Here's how the part is built. I have some questions about the finished solid (model axes, mm). A direction names the side the tool comes from. Coordinates: 2 decimals unless noted, no trailing zeros. Loops run counter-clockwise (first coordinate to the right, second up) from the corner with the lowest first, then second, coordinate; pieces in that order, holes last. Notation, with made-up numbers: (-28.5, 40) -> (22.5, 40) arc R31 ccw to (22.5, 79) -> close; hole circle Ø5 at (7.5, 23). An arc over 180 degrees is marked (long way). Answer as a JSON object with one key per item and string values. Group by question number.
Q1. I need wall thicknesses on line 1 (Z direction, x = -30.5, y = 95); line 2 (Z direction, x = 55, y = 8); line 3 (X direction, y = 60, z = 31.5). Which ranges of each line are inside material? Lowest first, please.
Q2. I want a section at C-C on z = 82.5. Write out the boundary of the cut face in (x, y).
Q3. I want a section at D-D on x = 43.5. Write out the boundary of the cut face in (y, z).
Q4. I'm going to push flat-ended pins straight in: pin 1 (0.8 mm diameter, centred on x = 24, z = 64, fed in from -Y); pin 2 (1.2 mm diameter, centred on x = 99.5, y = 43.5, fed in from +Z); pin 3 (1 mm diameter, centred on x = -36, y = 77, fed in from +Z); pin 4 (1 mm diameter, centred on x = 52, z = 55, fed in from +Y). Where does each tip first touch, or does it pass through?
Q5. On a 3-axis mill with a long thin cutter (end or side, diameter ignored), from which of +Z, -Z, +X, -X, +Y, -Y can I reach the whole of each face in a straight line? I mean faces 1 (the flat face through (-37, 94, 98.5)), 2 (the flat face through (-1, 0, -1)). Say none if no direction works.
Q6. Thinking about a two-plate mould opening in Y: for faces 3 (the flat face through (-100, 92, -2)), 4 (the flat face through (1.4, 149.375, -107.083)), 5 (the flat face through (61, 78, 30)), 6 (the flat face through (1.4, 169.1, -58)), which applies, released by +Y, released by -Y, zero draft, split by the parting line, or undercut?
Q7. I want a section at B-B on x = 71. Write out the boundary of the cut face in (y, z), then the cut area to 3 significant figures.
```python
from build123d import *

# Parameters (mm, degrees)
SKETCH_1_W           = 150
SKETCH_1_H           = 3.5
EXTRUDE_1_DEPTH      = 1.5
SKETCH_2_W           = 121.171669679
SKETCH_2_H           = 150
EXTRUDE_2_DEPTH      = 91.5
SKETCH_3_W           = 1.5
SKETCH_3_H           = 90
EXTRUDE_3_DEPTH      = 30
EXTRUDE_4_DEPTH      = 30
SKETCH_5_W           = 151.171669679
SKETCH_5_H           = 125
EXTRUDE_5_DEPTH      = 1.5
SKETCH_6_W           = 125
SKETCH_6_H           = 151.5
EXTRUDE_6_DEPTH      = 48.828330321
SKETCH_7_W           = 200
SKETCH_7_H           = 151.5
EXTRUDE_7_DEPTH      = 75
SKETCH_8_W           = 74.671669679
SKETCH_8_H           = 150
CUT_EXTRUDE_1_DEPTH  = 53.5
SKETCH_9_W           = 30
SKETCH_9_H           = 150
CUT_EXTRUDE_2_DEPTH  = 59.25
SKETCH_10_W          = 59.25
SKETCH_10_H          = 150
CUT_EXTRUDE_3_DEPTH  = 42.671669679
SKETCH_11_W          = 30
SKETCH_11_H          = 60
CUT_EXTRUDE_4_DEPTH  = 1.5
SKETCH_12_W          = 30
SKETCH_12_H          = 60
CUT_EXTRUDE_5_DEPTH  = 1.5
SKETCH_13_W          = 87
SKETCH_13_H          = 150
CUT_EXTRUDE_6_DEPTH  = 47.328330321
SKETCH_14_W          = 59.25
SKETCH_14_H          = 150
CUT_EXTRUDE_7_DEPTH  = 47.328330321
SKETCH_15_W          = 120
SKETCH_15_H          = 150
CUT_EXTRUDE_8_DEPTH  = 29.25
SKETCH_16_W          = 88.5
SKETCH_16_H          = 150
CUT_EXTRUDE_9_DEPTH  = 75.5
SKETCH_17_W          = 122
SKETCH_17_H          = 150
CUT_EXTRUDE_10_DEPTH = 20
SKETCH_18_W          = 50
SKETCH_18_H          = 150
CUT_EXTRUDE_11_DEPTH = 73.5
SKETCH_19_W          = 73.5
SKETCH_19_H          = 150
CUT_EXTRUDE_12_DEPTH = 18.5
SKETCH_20_W          = 75
SKETCH_20_H          = 150
CUT_EXTRUDE_13_DEPTH = 3.5
CUT_EXTRUDE_14_REACH = 272.097
SKETCH_21_W          = 30
SKETCH_21_H          = 30
CUT_EXTRUDE_15_REACH = 272.097
SKETCH_22_W          = 30
SKETCH_22_H          = 30
CUT_EXTRUDE_16_REACH = 272.097
SKETCH_23_W          = 30
SKETCH_23_H          = 30
EXTRUDE_11_DEPTH     = 200
EXTRUDE_12_DEPTH     = 200


with BuildPart() as part:
    # Sketch 1 → Extrude 1 (new body)
    with BuildSketch(Plane(origin=(98.5, 0, 0), x_dir=(0, -1, 0), z_dir=(-1, 0, 0))):
        with Locations((-76.5, -6.75)):
            Rectangle(SKETCH_1_W, SKETCH_1_H)
    extrude(amount=-EXTRUDE_1_DEPTH)

    # Sketch 2 → Extrude 2 (add)
    with BuildSketch(Plane(origin=(0, 0, -8.5), x_dir=(-1, 0, 0), z_dir=(0, 0, -1))):
        with Locations((-39.41416516, 76.5)):
            Rectangle(SKETCH_2_W, SKETCH_2_H)
    extrude(amount=EXTRUDE_2_DEPTH)

    # Sketch 3 → Extrude 3 (add)
    with BuildSketch(Plane.XY.offset(-5)):
        with Locations((99.25, 106.5)):
            Rectangle(SKETCH_3_W, SKETCH_3_H)
    extrude(amount=EXTRUDE_3_DEPTH)

    # Sketch 4 → Extrude 4 (add)
    with BuildSketch(Plane.ZY.offset(21.171669679)):
        Polygon((-100, 1.5), (-100, 151.5), (-8.5, 151.5), (-8.5, 61.5), (-10, 61.5), (-10, 1.5), align=None)
    extrude(amount=EXTRUDE_4_DEPTH)

    # Sketch 5 → Extrude 5 (add)
    with BuildSketch(Plane.XZ.offset(-1.5)):
        with Locations((24.41416516, -37.5)):
            Rectangle(SKETCH_5_W, SKETCH_5_H)
    extrude(amount=EXTRUDE_5_DEPTH)

    # Sketch 6 → Extrude 6 (add)
    with BuildSketch(Plane.ZY.offset(51.171669679)):
        with Locations((-37.5, 75.75)):
            Rectangle(SKETCH_6_W, SKETCH_6_H)
    extrude(amount=EXTRUDE_6_DEPTH)

    # Sketch 7 → Extrude 7 (add)
    with BuildSketch(Plane.XY.offset(25)):
        with Locations((0, 75.75)):
            Rectangle(SKETCH_7_W, SKETCH_7_H)
    extrude(amount=EXTRUDE_7_DEPTH)

    # Sketch 8 → Cut-Extrude 1 (cut)
    with BuildSketch(Plane(origin=(0, 0, 25), x_dir=(-1, 0, 0), z_dir=(0, 0, -1))):
        with Locations((13.83583484, 76.5)):
            Rectangle(SKETCH_8_W, SKETCH_8_H)
    extrude(amount=-CUT_EXTRUDE_1_DEPTH, mode=Mode.SUBTRACT)

    # Sketch 9 → Cut-Extrude 2 (cut)
    with BuildSketch(Plane.XY.offset(-10)):
        with Locations((-36.171669679, 76.5)):
            Rectangle(SKETCH_9_W, SKETCH_9_H)
    extrude(amount=-CUT_EXTRUDE_2_DEPTH, mode=Mode.SUBTRACT)

    # Sketch 10 → Cut-Extrude 3 (cut)
    with BuildSketch(Plane.ZY.offset(21.171669679)):
        with Locations((-39.625, 76.5)):
            Rectangle(SKETCH_10_W, SKETCH_10_H)
    extrude(amount=-CUT_EXTRUDE_3_DEPTH, mode=Mode.SUBTRACT)

    # Sketch 11 → Cut-Extrude 4 (cut)
    with BuildSketch(Plane.ZY.offset(-23.5)):
        with Locations((63.5, 31.5)):
            Rectangle(SKETCH_11_W, SKETCH_11_H)
    extrude(amount=-CUT_EXTRUDE_4_DEPTH, mode=Mode.SUBTRACT)

    # Sketch 12 → Cut-Extrude 5 (cut)
    with BuildSketch(Plane.ZY.offset(-21.5)):
        with Locations((-54.25, 31.5)):
            Rectangle(SKETCH_12_W, SKETCH_12_H)
    extrude(amount=-CUT_EXTRUDE_5_DEPTH, mode=Mode.SUBTRACT)

    # Sketch 13 → Cut-Extrude 6 (cut)
    with BuildSketch(Plane(origin=(-51.171669679, 0, 0), x_dir=(0, 0, -1), z_dir=(1, 0, 0))):
        with Locations((-35, 76.5)):
            Rectangle(SKETCH_13_W, SKETCH_13_H)
    extrude(amount=-CUT_EXTRUDE_6_DEPTH, mode=Mode.SUBTRACT)

    # Sketch 14 → Cut-Extrude 7 (cut)
    with BuildSketch(Plane(origin=(-51.171669679, 0, 0), x_dir=(0, 0, -1), z_dir=(1, 0, 0))):
        with Locations((39.625, 76.5)):
            Rectangle(SKETCH_14_W, SKETCH_14_H)
    extrude(amount=-CUT_EXTRUDE_7_DEPTH, mode=Mode.SUBTRACT)

    # Sketch 15 → Cut-Extrude 8 (cut)
    with BuildSketch(Plane.XY.offset(-69.25)):
        with Locations((-38.5, 76.5)):
            Rectangle(SKETCH_15_W, SKETCH_15_H)
    extrude(amount=-CUT_EXTRUDE_8_DEPTH, mode=Mode.SUBTRACT)

    # Sketch 16 → Cut-Extrude 9 (cut)
    with BuildSketch(Plane.ZY.offset(-23)):
        with Locations((-54.25, 76.5)):
            Rectangle(SKETCH_16_W, SKETCH_16_H)
    extrude(amount=-CUT_EXTRUDE_9_DEPTH, mode=Mode.SUBTRACT)

    # Sketch 17 → Cut-Extrude 10 (cut)
    with BuildSketch(Plane(origin=(0, 0, 78.5), x_dir=(-1, 0, 0), z_dir=(0, 0, -1))):
        with Locations((37.5, 76.5)):
            Rectangle(SKETCH_17_W, SKETCH_17_H)
    extrude(amount=-CUT_EXTRUDE_10_DEPTH, mode=Mode.SUBTRACT)

    # Sketch 18 → Cut-Extrude 11 (cut)
    with BuildSketch(Plane.ZY.offset(-25)):
        with Locations((73.5, 76.5)):
            Rectangle(SKETCH_18_W, SKETCH_18_H)
    extrude(amount=-CUT_EXTRUDE_11_DEPTH, mode=Mode.SUBTRACT)

    # Sketch 19 → Cut-Extrude 12 (cut)
    with BuildSketch(Plane.XY.offset(48.5)):
        with Locations((61.75, 76.5)):
            Rectangle(SKETCH_19_W, SKETCH_19_H)
    extrude(amount=-CUT_EXTRUDE_12_DEPTH, mode=Mode.SUBTRACT)

    # Sketch 20 → Cut-Extrude 13 (cut)
    with BuildSketch(Plane(origin=(0, 0, 25), x_dir=(-1, 0, 0), z_dir=(0, 0, -1))):
        with Locations((-61, 76.5)):
            Rectangle(SKETCH_20_W, SKETCH_20_H)
    extrude(amount=-CUT_EXTRUDE_13_DEPTH, mode=Mode.SUBTRACT)

    # Sketch 21 → Cut-Extrude 14 (cut, up to next)
    with BuildSketch(Plane(origin=(0, 0, -100), x_dir=(-1, 0, 0), z_dir=(0, 0, -1)), mode=Mode.PRIVATE) as cut_extrude_14_sk1:
        with Locations((-52.804007689, 60.155834385)):
            Rectangle(SKETCH_21_W, SKETCH_21_H)
    cut_extrude_14_tool1 = extrude(cut_extrude_14_sk1.sketch, amount=-CUT_EXTRUDE_14_REACH, mode=Mode.PRIVATE) & part.part
    add(cut_extrude_14_tool1.solids().sort_by_distance((52.804008, 60.155834, -100))[0], mode=Mode.SUBTRACT)

    # Sketch 22 → Cut-Extrude 15 (cut, up to next)
    with BuildSketch(Plane(origin=(0, 0, -100), x_dir=(-1, 0, 0), z_dir=(0, 0, -1)), mode=Mode.PRIVATE) as cut_extrude_15_sk1:
        with Locations((36.226594007, 60.594472186)):
            Rectangle(SKETCH_22_W, SKETCH_22_H)
    cut_extrude_15_tool1 = extrude(cut_extrude_15_sk1.sketch, amount=-CUT_EXTRUDE_15_REACH, mode=Mode.PRIVATE) & part.part
    add(cut_extrude_15_tool1.solids().sort_by_distance((-36.226594, 60.594472, -100))[0], mode=Mode.SUBTRACT)

    # Sketch 23 → Cut-Extrude 16 (cut, up to next)
    with BuildSketch(Plane.XY.offset(100), mode=Mode.PRIVATE) as cut_extrude_16_sk1:
        with Locations((-38.061358281, 75.75)):
            Rectangle(SKETCH_23_W, SKETCH_23_H)
    cut_extrude_16_tool1 = extrude(cut_extrude_16_sk1.sketch, amount=-CUT_EXTRUDE_16_REACH, mode=Mode.PRIVATE) & part.part
    add(cut_extrude_16_tool1.solids().sort_by_distance((-38.061358, 75.75, 100))[0], mode=Mode.SUBTRACT)



with BuildPart() as body_2:
    # Sketch 26 → Extrude 11 (new body)
    with BuildSketch(Plane(origin=(100, 0, 0), x_dir=(0, 0, -1), z_dir=(1, 0, 0))):
        Polygon((-100, 151.5), (0, 181.5), (100, 151.5), (114.367394278, 147.189781717), (114.367394278, 152.189781717), (0, 186.5), (-114.367394278, 152.189781717), (-114.367394278, 147.189781717), align=None)
    extrude(amount=-EXTRUDE_11_DEPTH)


with BuildPart() as part_1:
    add(part.part)

    add(body_2.part)  # Extrude 12 merges body 2
    # Sketch 27 → Extrude 12 (add)
    with BuildSketch(Plane(origin=(100, 0, 0), x_dir=(0, 0, -1), z_dir=(1, 0, 0))):
        Polygon((0, 181.5), (-100, 151.5), (0, 151.5), (100, 151.5), align=None)
    extrude(amount=-EXTRUDE_12_DEPTH)


solid = part_1.part
```
Result set:
{
 "1": {"line 1": "z = -100 to -98.5, -10 to -8.5, 98.5 to 100", "line 2": "z = -100 to -98.5, -10 to -8.5, 28.5 to 30, 98.5 to 100", "line 3": "x = -100 to -98.5, 23.5 to 25, 98.5 to 100"},
 "2": {"outline": "(-100, 0) -> (100, 0) -> (100, 161.75) -> (-100, 161.75) -> close; hole (-98.5, 1.5) -> (23.5, 1.5) -> (23.5, 151.5) -> (-98.5, 151.5) -> close; hole (25, 1.5) -> (98.5, 1.5) -> (98.5, 151.5) -> (25, 151.5) -> close"},
 "3": {"outline": "(0, -100) -> (45.16, -100) -> (45.16, -98.5) -> (1.5, -98.5) -> (1.5, -10) -> (151.5, -10) -> (151.5, -98.5) -> (75.16, -98.5) -> (75.16, -100) -> (151.5, -100) -> (147.19, -114.37) -> (152.19, -114.37) -> (186.5, 0) -> (152.19, 114.37) -> (147.19, 114.37) -> (151.5, 100) -> (0, 100) -> close; hole (1.5, -8.5) -> (151.5, -8.5) -> (151.5, 28.5) -> (1.5, 28.5) -> close; hole (1.5, 30) -> (151.5, 30) -> (151.5, 98.5) -> (1.5, 98.5) -> close"},
 "4": {"pin 1": "stops at y = 0", "pin 2": "stops at z = 100", "pin 3": "stops at z = -8.5", "pin 4": "stops at y = 170.15"},
 "5": {"face 1": "none", "face 2": "+Z, -Z, +X, -X, -Y"},
 "6": {"face 3": "zero draft", "face 4": "released by -Y", "face 5": "undercut", "face 6": "released by +Y"},
 "7": {"outline": "(0, -100) -> (151.5, -100) -> (147.19, -114.37) -> (152.19, -114.37) -> (186.5, 0) -> (152.19, 114.37) -> (147.19, 114.37) -> (151.5, 100) -> (0, 100) -> close; hole (1.5, -98.5) -> (151.5, -98.5) -> (151.5, -10) -> (1.5, -10) -> close; hole (1.5, -8.5) -> (151.5, -8.5) -> (151.5, 28.5) -> (1.5, 28.5) -> close; hole (1.5, 30) -> (151.5, 30) -> (151.5, 98.5) -> (1.5, 98.5) -> close", "area": "5,340 mm²"}
}
